```python
from build123d import *

# Parameters (mm, degrees)
SKETCH1_R           = 3.75
BOSS_EXTRUDE1_DEPTH = 12
SKETCH2_R           = 1.75
CUT_EXTRUDE1_DEPTH  = 16


with BuildPart() as part:
    # Sketch1 → Boss-Extrude1 (new body)
    with BuildSketch(Plane(origin=(0, 0, 0), x_dir=(0, 0, -1), z_dir=(1, 0, 0))):
        Polygon((-7.5, 20), (-3.5, 20), (-3.5, 13), (3.5, 13), (3.5, 20), (7.5, 20), (7.5, -20), (3.5, -20), (3.5, -13), (-3.5, -13), (-3.5, -20), (-7.5, -20), align=None)
        Circle(SKETCH1_R, mode=Mode.SUBTRACT)
    extrude(amount=BOSS_EXTRUDE1_DEPTH)

    # Sketch2 → Cut-Extrude1 (cut, through all)
    with BuildSketch(Plane.XY.offset(7.5)):
        with BuildLine():
            ThreePointArc((1.301959033, 14.335379208), (0.344469259, 15.447503856), (0, 16.874020182))
            Line((0, 16.874020182), (0, -16.874020197))
            ThreePointArc((0, -16.874020197), (0.344469255, -15.447503862), (1.301959033, -14.335379208))
            Line((1.301959033, -14.335379208), (6.934312509, -10.288517163))
            Line((6.934312509, -10.288517163), (6.934312509, 10.288517163))
            Line((6.934312509, 10.288517163), (1.301959033, 14.335379208))
        make_face()
        with BuildLine():
            ThreePointArc((0, 16.874020182), (0.915578291, 19.084421709), (3.125979818, 20))
            Line((3.125979818, 20), (0, 20))
            Line((0, 20), (0, 16.874020182))
        make_face()
        with Locations((3.125979818, 16.874020182)):
            Circle(SKETCH2_R)
        with BuildLine():
            ThreePointArc((3.125979818, 20), (4.251738736, 19.790253486), (5.226425655, 19.189161021))
            Line((5.226425655, 19.189161021), (8.613212827, 16.116448166))
            Line((8.613212827, 16.116448166), (12, 13.043735311))
            Line((12, 13.043735311), (12, 20))
            Line((12, 20), (3.125979818, 20))
        make_face()
        with BuildLine():
            Line((12, -20), (12, -13.043735311))
            Line((12, -13.043735311), (8.613212827, -16.116448166))
            Line((8.613212827, -16.116448166), (5.226425655, -19.189161021))
            ThreePointArc((5.226425655, -19.189161021), (4.251738736, -19.790253486), (3.125979818, -20))
            Line((3.125979818, -20), (12, -20))
        make_face()
        with BuildLine():
            ThreePointArc((3.125979818, -20), (0.915578296, -19.084421715), (0, -16.874020197))
            Line((0, -16.874020197), (0, -20))
            Line((0, -20), (3.125979818, -20))
        make_face()
        with Locations((3.125979818, -16.874020182)):
            Circle(SKETCH2_R)
    extrude(amount=-CUT_EXTRUDE1_DEPTH, mode=Mode.SUBTRACT)


solid = part.part
```
Part model, mm, in its own coordinate system. A direction names the side the tool comes from. Give positions to 0.01 mm unless a question says otherwise; leave off trailing zeros. Order: outer loops, then holes, each group sorted by start corner. A loop starts at its lowest first (then second) coordinate and runs counter-clockwise, first axis right, second up. Notation, with made-up numbers: (21, -9.75) - (46, -9.75) arc R27 cw to (46, 10.25) - close; hole circle Ø3 at (83, 54.5). An arc over 180 degrees is marked (long way). Use one line per item in the form item = value.
Item 1: Which spindle directions (+Z, -Z, +X, -X, +Y, -Y) get a long thin tool onto all of the face, cutting with end or side? Do faces 1 (the face through (5, -16, -3.5)), 2 (the face through (6, 16, -3.5)), 3 (the face through (4.705, -11.891, 0.105)). Say none if no direction does.
Solution:
face_1 = +X, -X, -Y
face_2 = +X, -X, +Y
face_3 = +Z, -Z, -X
Item 2: Slice it at A-A on y = 0. Give the cut face in (x, z), and give its area (3 significant figures).
Solution:
outline = (6.93, -7.5) - (12, -7.5) - (12, -3.75) - (6.93, -3.75) - close; (6.93, 3.75) - (12, 3.75) - (12, 7.5) - (6.93, 7.5) - close
area = 38.0 mm2
Item 3: Slice it at B-B on z = -3. Give the cut face in (x, y), and give its area (3 significant figures).
Solution:
outline = (3.16, -13) - (12, -13) - (12, -2.25) - (6.93, -2.25) - (6.93, -10.29) - close; (3.16, 13) - (6.93, 10.29) - (6.93, 2.25) - (12, 2.25) - (12, 13) - close
area = 119 mm2
Item 4: Slice it at D-D on z = 0. Give the cut face in (x, y), and give its area (3 significant figures).
Solution:
outline = (3.16, -13) - (12, -13) - (12, -3.75) - (6.93, -3.75) - (6.93, -10.29) - close; (3.16, 13) - (6.93, 10.29) - (6.93, 3.75) - (12, 3.75) - (12, 13) - close
area = 104 mm2
Item 5: Two-plate mould, pull along Y, no slides. Class faces 4 (the face through (8, 13, 0)), 5 (the face through (6, -16, 3.5)), 6 (the face through (8, -13, 0)), 7 (the face through (4.783, 11.834, 0.105)): released by +Y, released by -Y, zero draft, split by the parting line, or undercut.
Solution:
face_4 = released by +Y
face_5 = zero draft
face_6 = released by -Y
face_7 = undercut
Item 6: Slice it at C-C on x = 6. Give the cut face in (y, z), and give its area (3 significant figures).
Solution:
outline = (-18.49, -7.5) - (-10.96, -7.5) - (-10.96, 7.5) - (-18.49, 7.5) - (-18.49, 3.5) - (-13, 3.5) - (-13, -3.5) - (-18.49, -3.5) - close; (10.96, -7.5) - (18.49, -7.5) - (18.49, -3.5) - (13, -3.5) - (13, 3.5) - (18.49, 3.5) - (18.49, 7.5) - (10.96, 7.5) - close
area = 149 mm2
Item 7: Probe probe 1 along Y at (x, z) = (8.2, 0); probe 2 along Z at (x, y) = (6, -16); probe 3 along Y at (x, z) = (2, -4). List the from-to ranges inside material, lowest first. Write a range as from..to.
Solution:
probe_1 = -13..-3.75, 3.75..13
probe_2 = -7.5..-3.5, 3.5..7.5
probe_3 = -19.79..-18.21, -15.53..-13.83, 13.83..15.53, 18.21..19.79
Item 8: Pin check, flat tips, straight feed: pin 1 Ø4.5 at (y, z) = (5, 0) entering from -X; pin 2 Ø3 at (x, y) = (3.13, 16.87) entering from +Z; pin 3 Ø1 at (x, z) = (7.5, -2) entering from +Y; pin 4 Ø1 at (x, z) = (3.5, 2) entering from -Y. Stop position of each tip, or through.
Solution:
pin_1 = 6.93
pin_2 = through
pin_3 = 13
pin_4 = -13
